For this review, take the finished solid that the model builds, in its own axes (mm). Face numbers are marked on the shaded views. Give positions to 0.01 mm unless a question says otherwise; leave off trailing zeros. Order: outer loops, then holes, each group sorted by start corner. A loop starts at its lowest first (then second) coordinate and runs counter-clockwise, first axis right, second up. Notation, with made-up numbers: M 21.25,11.5 L 73.25,11.5 A11 ccw 73.25,27.5 Z; hole C -9,-21 d6. An arc over 180 degrees is marked long. Use CSV: the item, a comma, the result in double quotes. Start each with the question number.
(1) Clearance check with flat-ended pins moving along their axes: P1, Ø2, axis at x = 3.5, z = 14, coming from the +Y side; P2, Ø1, axis at x = 5.5, y = 13.5, coming from the +Z side; P3, Ø4, axis at x = 4, y = -14, coming from the +Z side. State where each tip first meets the part, or that it passes through.
(2) Draft analysis for pull direction Z (two halves, no side actions). For the marked faces 1, 2 and 3, state which applies: pulls with the +Z half, pulls with the -Z half, needs draft (parallel to the pull), parting line crosses it, or undercut.
(3) Wall thickness on L1, parallel to Y at x = 4.75, z = 0; L2, parallel to Z at x = 7, y = -3; L3, parallel to Y at x = 7.5, z = -1: over which ranges is each line inside the solid? List them lowest first. Write a range as from..to.
(4) Consider section A-A (y = 0). Write out the cut boundary in (x, z).
(5) Consider section B-B (x = 6.5). Write out the cut boundary in (y, z).
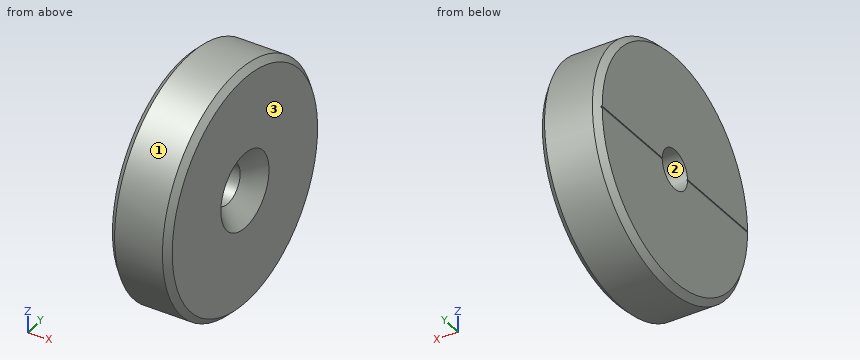
```python
from build123d import *

# Parameters (mm, degrees)
ESQUISSE1_W             = 10
ESQUISSE1_H             = 20
CHANFREIN1_SIZE         = 1
PER_AGE1_D              = 6.6
PER_AGE1_CSINK_D        = 12.6
PER_AGE1_CSINK_ANGLE    = 92
ESQUISSE5_W             = 2.1
ESQUISSE5_H             = 0.25
ENL_V_MAT_EXTRU_1_DEPTH = 20


with BuildPart() as part:
    # Esquisse1 → Base-Révolution (revolve)
    with BuildSketch(Plane.XY, mode=Mode.PRIVATE) as base_r_volution_sk:
        with Locations((5, 10)):
            Rectangle(ESQUISSE1_W, ESQUISSE1_H)
    revolve(base_r_volution_sk.sketch.rotate(Axis((0, 0, 0), (1, 0, 0)), 90), axis=Axis((0, 0, 0), (1, 0, 0)))

    # Chanfrein1
    chanfrein1_edges = [part.edges().sort_by_distance(p)[0] for p in [
        (10, 0, -20),
        (0, 0, -20),
    ]]
    chamfer(chanfrein1_edges, length=CHANFREIN1_SIZE)

    # Perçage1 (through all)
    with Locations(Plane(origin=(10, 0, 0), x_dir=(0, 0, -1), z_dir=(1, 0, 0))):
        with Locations((0, 0)):
            CounterSinkHole(PER_AGE1_D / 2, PER_AGE1_CSINK_D / 2, counter_sink_angle=PER_AGE1_CSINK_ANGLE)

    # Esquisse5 → Enlèv. mat.-Extru.1 (cut, symmetric)
    with BuildSketch(Plane(origin=(0, 0, 0), x_dir=(1, 0, 0), z_dir=(0, 1, 0))):
        with Locations((-0.95, 0)):
            Rectangle(ESQUISSE5_W, ESQUISSE5_H)
    extrude(amount=ENL_V_MAT_EXTRU_1_DEPTH, both=True, mode=Mode.SUBTRACT)


solid = part.part
```
Check result:
1,P1,"stops at y = 15.2"
1,P2,"stops at z = 15.2"
1,P3,"stops at z = 16"
2,face 1,"parting line crosses it"
2,face 2,"undercut"
2,face 3,"needs draft"
3,L1,"y = -20..-3.3, 3.3..20"
3,L2,"z = -19.77..-1.37, 1.37..19.77"
3,L3,"y = -19.97..-3.57, 3.57..19.97"
4,outline,"M 0,-19 L 1,-20 L 9,-20 L 10,-19 L 10,-6.3 L 7.1,-3.3 L 0,-3.3 Z; M 0,3.3 L 7.1,3.3 L 10,6.3 L 10,19 L 9,20 L 1,20 L 0,19 Z"
5,outline,"C 0,0 d40; hole C 0,0 d6.6"
